Can you work these out from the drawing? Everything is in mm from the part's minimum corner. Give positions to 0.01 mm unless a question says otherwise; leave off trailing zeros. Loops run counter-clockwise (first coordinate to the right, second up) from the corner with the lowest first, then second, coordinate; pieces in that order, holes last.
Q1. I need wall thicknesses on line 1 (Y direction, x = 19.65, z = 3.5); line 2 (Y direction, x = 107.35, z = 9); line 3 (X direction, y = 115, z = 9). Which ranges of each line are inside material? Lowest first, please.
Q2. Will this pin go through, and if not, where does the flat tip stop? P1, Ø8, axis at x = 19.65, y = 97.6, coming from the -Z side.
Q3. If we section it at A-A (y = 97.6): Please give me the cut outline in (x, z), plus the area to 3 significant figures.
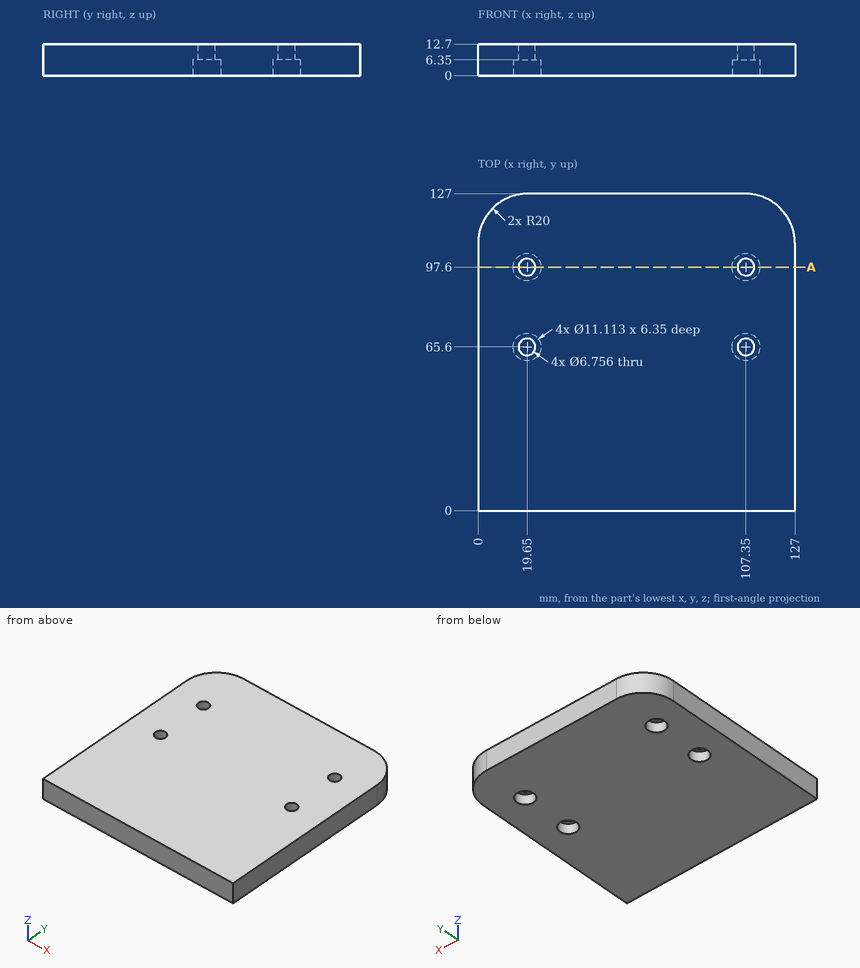
Check sheet entries:
1. line 1: y = 0 to 60.04, 71.16 to 92.04, 103.16 to 127
1. line 2: y = 0 to 62.22, 68.98 to 94.22, 100.98 to 127
1. line 3: x = 1.67 to 125.33
2. P1: stops at z = 6.35
3. outline: (0, 0) - (14.09, 0) - (14.09, 6.35) - (16.27, 6.35) - (16.27, 12.7) - (0, 12.7) - close; (23.03, 6.35) - (25.21, 6.35) - (25.21, 0) - (101.79, 0) - (101.79, 6.35) - (103.97, 6.35) - (103.97, 12.7) - (23.03, 12.7) - close; (110.73, 6.35) - (112.91, 6.35) - (112.91, 0) - (127, 0) - (127, 12.7) - (110.73, 12.7) - close
3. area: 1,390 mm2
